Part model, mm, in its own coordinate system. A direction names the side the tool comes from. Give positions to 0.01 mm unless a question says otherwise; leave off trailing zeros. Order: outer loops, then holes, each group sorted by start corner. A loop starts at its lowest first (then second) coordinate and runs counter-clockwise, first axis right, second up. Notation, with made-up numbers: (-20.75, 9.5) - (-11.75, 9.5) arc R27 ccw to (-11.75, 38.5) - close; hole circle Ø2 at (61, -19.5). An arc over 180 degrees is marked (long way). One line per item, written item: value.
```python
from build123d import *

# Parameters (mm, degrees)
SKETCH_W             = 70
SKETCH_H             = 40
PAD_DEPTH            = 8
POCKET_DEPTH         = 4
SKETCH002_R          = 2
POCKET001_DEPTH      = 4.001
SKETCH003_W          = 64.25
SKETCH003_H          = 24
POCKET002_DEPTH      = 4
SKETCH004_R          = 2
POCKET003_DEPTH      = 4
SKETCH005_W          = 35
SKETCH005_H          = 12
POCKET004_DEPTH      = 4
POCKET005_DEPTH      = 8.001
SKETCH009_W          = 5.75
SKETCH009_H          = 15
POCKET006_DEPTH      = 1.5
FILLET_R             = 2.75
CHAMFER_SIZE         = 1
BODY_PLACEMENT_ANGLE = 90


with BuildPart() as part:
    # Sketch → Pad (new body)
    with BuildSketch(Plane.XZ):
        Rectangle(SKETCH_W, SKETCH_H)
    extrude(amount=PAD_DEPTH)

    # Sketch001 (on Face5 of Pad) → Pocket (cut)
    with BuildSketch(Plane(origin=(0, 0, 0), x_dir=(1, 0, 0), z_dir=(0, 1, 0))):
        with BuildLine():
            Line((31.8, -20), (31.8, -7))
            ThreePointArc((31.8, -7), (31.507107, -6.292893), (30.8, -6))
            Line((30.8, -6), (-9.2, -6))
            ThreePointArc((-9.2, -6), (-9.907107, -6.292893), (-10.2, -7))
            Line((-10.2, -7), (-10.2, -20))
            Line((-10.2, -20), (31.8, -20))
        make_face()
    extrude(amount=-POCKET_DEPTH, mode=Mode.SUBTRACT)

    # Sketch002 (on Face7 of Pocket) → Pocket001 (cut, through all)
    with BuildSketch(Plane(origin=(0, -4, 0), x_dir=(1, 0, 0), z_dir=(0, 1, 0))):
        with Locations((-4.825, -11.78)):
            Circle(SKETCH002_R)
        with Locations((26.425, -11.78)):
            Circle(SKETCH002_R)
    extrude(amount=-POCKET001_DEPTH, mode=Mode.SUBTRACT)

    # Sketch003 (on Face5 of Pocket001) → Pocket002 (cut)
    with BuildSketch(Plane.XZ.offset(8)):
        with Locations((-2.875, -8)):
            Rectangle(SKETCH003_W, SKETCH003_H)
    extrude(amount=-POCKET002_DEPTH, mode=Mode.SUBTRACT)

    # Sketch004 (on Face4 of Pocket002) → Pocket003 (cut)
    with BuildSketch(Plane.XZ.offset(4)):
        with Locations((14.9, -3.25)):
            Circle(SKETCH004_R)
        with Locations((-31.5, -6.25)):
            Circle(SKETCH004_R)
    extrude(amount=-POCKET003_DEPTH, mode=Mode.SUBTRACT)

    # Sketch005 (on Face4 of Pocket003) → Pocket004 (cut)
    with BuildSketch(Plane.XZ.offset(4)):
        with Locations((5.5, -14)):
            Rectangle(SKETCH005_W, SKETCH005_H)
    extrude(amount=-POCKET004_DEPTH, mode=Mode.SUBTRACT)

    # Sketch008 (on Face2 of Pocket004) → Pocket005 (cut, through all)
    with BuildSketch(Plane(origin=(0, 0, 0), x_dir=(1, 0, 0), z_dir=(0, 1, 0))):
        with BuildLine():
            ThreePointArc((-7.5, 6), (-4.5, 3), (-1.5, 6))
            Line((-1.5, 8), (-1.5, 6))
            Line((-7.5, 8), (-1.5, 8))
            Line((-7.5, 8), (-7.5, 6))
        make_face()
    extrude(amount=-POCKET005_DEPTH, mode=Mode.SUBTRACT)

    # Sketch009 (on Face6 of Pocket005) → Pocket006 (cut)
    with BuildSketch(Plane.XZ.offset(8)):
        with BuildLine():
            Line((-35, 4), (5, 4))
            Line((5, 4), (5, 8.5))
            ThreePointArc((5, 8.5), (4.707107, 9.207107), (4, 9.5))
            Line((4, 9.5), (-35, 9.5))
            Line((-35, 9.5), (-35, 4))
        make_face()
        with Locations((32.125, -12.5)):
            Rectangle(SKETCH009_W, SKETCH009_H)
    extrude(amount=-POCKET006_DEPTH, mode=Mode.SUBTRACT)

    # Fillet
    fillet_edges = [part.edges().sort_by_distance(p)[0] for p in [
        (35, -4, 20),
        (-35, -4, 20),
        (35, -3.25, -20),
        (-35, -2, -20),
    ]]
    fillet(fillet_edges, radius=FILLET_R)

    # Chamfer
    chamfer_edges = [part.edges().sort_by_distance(p)[0] for p in [
        (-10.2, -2, 20),
    ]]
    chamfer(chamfer_edges, length=CHAMFER_SIZE)


with BuildPart() as part_1:
    # Body placement: moved
    add(part.part.rotate(Axis((0, 0, 0), (-1, 0, 0)), BODY_PLACEMENT_ANGLE))


solid = part_1.part
```
1) Mould opens along X. For faces 4 (the cylindrical face through (-5.1, 9.8, 6)), 5 (the flat face through (-15, 7, 6.5)), 6 (the flat face through (11, 6, 2)), 7 (the flat face through (-35, 4, 3)) say: released by +X, released by -X, zero draft, split by the parting line, or undercut.
Outcome:
face 4: undercut
face 5: zero draft
face 6: undercut
face 7: released by -X
2) Which spindle directions (+Z, -Z, +X, -X, +Y, -Y) get a long thin tool onto all of the face, cutting with end or side? Do faces 1 (the flat face through (-3, 4, 6)), 2 (the flat face through (-10.2, 13, 2)), 3 (the flat face through (-12, -14, 2)). Say none if no direction does.
Outcome:
face 1: +Z, -X, -Y
face 2: -Z, +Y
face 3: +Z, -Z, -Y
3) Drill centre lines: line 1 along X through (y, z) = (11.78, 4.8) (3 decimals); line 2 along X through (y, z) = (15, 3.5); line 3 along Y through (x, z) = (-31.5, 2.3). Where is each one in solid material? Low to high. Write a range as from..to.
Outcome:
line 1: x = -35..-6.825, -2.825..24.425, 28.425..35
line 2: x = -35..-10.2, 31.8..35
line 3: y = -20..-8.25, -4.25..20
4) Cut at D-D, the plane y = 2. Give the cut face in (x, z), then the cut area to 3 significant figures.
Outcome:
outline: (-35, 0) - (35, 0) - (35, 8) - (29.25, 8) - (29.25, 4) - (-35, 4) - close
area: 303 mm^2
5) Cut at A-A, the plane x = 14.9. Give the cut face in (y, z).
Outcome:
outline: (-8, 0) - (-5.25, 0) - (-5.25, 4) - (-8, 4) - close; (-1.25, 0) - (6, 0) - (6, 4) - (20, 4) - (20, 8) - (4, 8) - (4, 4) - (-1.25, 4) - close
6) Cut at C-C, the plane y = 11.78. Give the cut face in (x, z) (3 decimals), then the cut area to 3 significant figures.
Outcome:
outline: (-35, 0) - (-10.2, 0) - (-10.2, 4) - (-6.825, 4) - (-6.825, 8) - (-35, 8) - close; (-2.825, 4) - (24.425, 4) - (24.425, 8) - (-2.825, 8) - close; (28.425, 4) - (31.8, 4) - (31.8, 0) - (35, 0) - (35, 8) - (28.425, 8) - close
area: 360 mm^2
7) Cut at B-B, the plane z = 2.75. Give the cut face in (x, y).
Outcome:
outline: (-35, -17.25) arc R2.75 ccw to (-32.25, -20) - (-12, -20) - (-12, -8) - (-7.5, -8) - (-7.5, -6) arc R3 cw to (-1.5, -6) - (-1.5, -8) - (23, -8) - (23, -20) - (32.25, -20) arc R2.75 ccw to (35, -17.25) - (35, 17.25) arc R2.75 ccw to (32.25, 20) - (31.8, 20) - (31.8, 7) arc R1 cw to (30.8, 6) - (-9.2, 6) arc R1 cw to (-10.2, 7) - (-10.2, 19) - (-11.2, 20) - (-32.25, 20) arc R2.75 ccw to (-35, 17.25) - close; hole circle Ø4 at (-31.5, -6.25); hole circle Ø4 at (14.9, -3.25)
8) Pin check, flat tips, straight feed: pin 1 (1.2 mm diameter, centred on x = -10.5, z = 2.5, fed in from -Y); pin 2 (5 mm diameter, centred on x = -4.825, y = 11.78, fed in from -Z); pin 3 (3 mm diameter, centred on x = -5, y = 7.5, fed in from +Z). Stop position of each tip, or through.
Outcome:
pin 1: stops at y = -8
pin 2: stops at z = 4
pin 3: stops at z = 6.5
